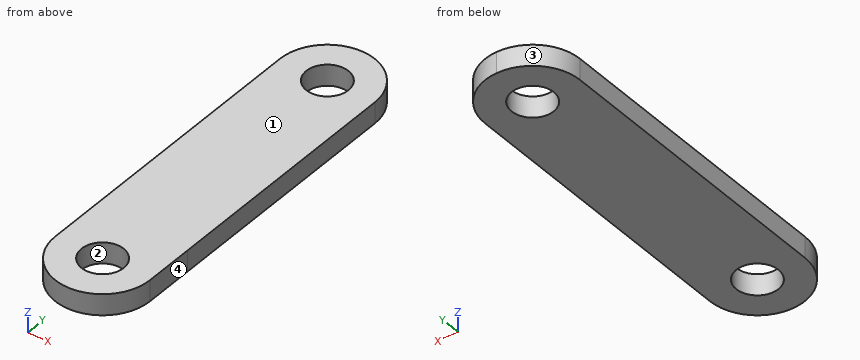
Autodesk Inventor part; units mm, degrees
ref_plane "Work Plane1" through (0, 0, 3.5) normal (0, 0, 1) x (1, 0, 0)
ref_plane "YZ Plane" through (0, 0, 0) normal (1, 0, 0) x (0, 1, 0)
ref_plane "XZ Plane" through (0, 0, 0) normal (0, 1, 0) x (-1, 0, 0)
ref_plane "Work Plane1" through (0, 0, 3.5) normal (0, 0, 1) x (1, 0, 0)
sketch "Sketch2" plane through (0, 0, 3.5) normal (0, 0, 1) x (1, 0, 0)
  circle A0 centre (0, 0) radius 13
  line L0 (13, 0) -> (-13, 0)
  line L1 (-13, 0) -> (-13, 65)
  line L2 (-13, 65) -> (13, 65)
  line L3 (13, 65) -> (13, 0)
  line L4 (9, 0) -> (-9, 0)
  line L5 (-9, 0) -> (-9, 65)
  line L6 (-9, 65) -> (9, 65)
  line L7 (9, 65) -> (9, 0)
  point P0 (9, 9.3808)
  point P1 (9, 65)
  point P2 (-9, 9.3808)
  dimension "d5" = 65
  dimension "d15" = 18
extrude "Extrusion2" add sketch "Sketch2" along normal blind 2 and the other way blind 2 contours L5 L2 L7 A0
fillet "Fillet1" radius 9 2 edges at (9, 65, 3.5) (-9, 65, 3.5)
sketch "Sketch3" plane through (0, 0, 5.5) normal (0, 0, 1) x (1, 0, 0)
  circle A0 centre (0, 56) radius 4
  arc A1 (9, 56) -> (-9, 56) centre (0, 56) ccw
  point P0 (0, 0)
  dimension "d11" = 8
  dimension "d17" = 0
extrude "Extrusion3" cut sketch "Sketch3" against normal up to surface (4 mm away)
sketch "Sketch4" plane through (0, 0, 5.5) normal (0, 0, 1) x (1, 0, 0)
  circle A0 centre (0, 0) radius 11
  circle A1 centre (0, 0) radius 4
  circle A2 centre (0, 0) radius 9
  line L0 (9, 9.3808) -> (9, 56)
  line L1 (9, 0) -> (9, 9.3808)
  line L2 (-9, 0) -> (-9, 9.8723)
  line L3 (-9, 56) -> (-9, 9.3808)
  line L4 (9, 9.3808) -> (4, 16.3545)
  line L5 (4, 16.3545) -> (-2.5597, 14.9818)
  line L6 (-2.5597, 14.9818) -> (-9, 9.8723)
  dimension "d18" = 8
  dimension "d19" = 18
extrude "Extrusion4" add sketch "Sketch4" against normal blind 4 contours L1 A2 L2 A0 | A0 L2 L6 L5 L4 L1 | A2 picked at (7.6596, 6.8574)
properties part number "zawieszenie ramie"
Check sheet for the modelled part. Datum: model origin and axes. Units: mm. Face numbers are marked on the shaded views. Coordinates: 2 decimals unless noted, no trailing zeros. Loops run counter-clockwise (first coordinate to the right, second up) from the corner with the lowest first, then second, coordinate; pieces in that order, holes last. Notation, with made-up numbers: (9, -37.75) -> (66, -37.75) arc R22 cw to (66, -1.75) -> close; hole circle Ø11 at (84, -21). An arc over 180 degrees is marked (long way). Answer in a Markdown table with one row per item.
1. Go/stop test with a flat-tipped pin: pin 1 (1 mm diameter, centred on x = 2.5, y = 57.5, fed in from -Z). Record where the tip stops, or that it passes through.
Check values:
| item | result |
|---|---|
| pin 1 | passes through |
2. Sectioned sample at A-A, the plane z = 4.6. Give the number of separate pieces and of enclosed holes in the cut face, then the cut area to 3 significant figures.
Check values:
| item | result |
|---|---|
| separate pieces | 1 |
| enclosed holes | 2 |
| area | 1,160 mm2 |
3. Sectioned sample at C-C, the plane y = 2. Record the boundary of the cut face in (x, z), then the cut area to 3 significant figures.
Check values:
| item | result |
|---|---|
| outline | (-9, 1.5) -> (-3.46, 1.5) -> (-3.46, 5.5) -> (-9, 5.5) -> close; (3.46, 1.5) -> (9, 1.5) -> (9, 5.5) -> (3.46, 5.5) -> close |
| area | 44.3 mm2 |
4. Material ranges on line 1 along Y through (x, z) = (0, 3.9); line 2 along X through (y, z) = (55, 3.6); line 3 along Y through (x, z) = (6.5, 3), recorded low to high. Write a range as [from, to].
Check values:
| item | result |
|---|---|
| line 1 | y = [-9, -4], [4, 52], [60, 65] |
| line 2 | x = [-9, -3.87], [3.87, 9] |
| line 3 | y = [-6.22, 62.23] |
5. Release check for a two-part mould opening along X. For the marked faces 1, 2, 3 and 4 record: released by +X, released by -X, zero draft, split by the parting line, or undercut.
Check values:
| item | result |
|---|---|
| face 1 | zero draft |
| face 2 | undercut |
| face 3 | released by -X |
| face 4 | released by +X |
6. Sectioned sample at B-B, the plane x = 1.25. Record the boundary of the cut face in (y, z).
Check values:
| item | result |
|---|---|
| outline | (-8.91, 1.5) -> (-3.8, 1.5) -> (-3.8, 5.5) -> (-8.91, 5.5) -> close; (3.8, 1.5) -> (52.2, 1.5) -> (52.2, 5.5) -> (3.8, 5.5) -> close; (59.8, 1.5) -> (64.91, 1.5) -> (64.91, 5.5) -> (59.8, 5.5) -> close |
